```python
from build123d import *

# Parameters (mm, degrees)
F0_R     = 1.9
F0_W     = 19.35
F0_H     = 8
F0_R_2   = 1
F1_DEPTH = 8
F2_R     = 2


with BuildPart() as f1:
    # F0 (on Top) → F1 (new body)
    with BuildSketch(Plane.XY):
        Polygon((50, 22.5), (0, 22.5), (0, 0), (14.45, 0), (33.8, 0), (50, 0), align=None)
        with Locations((7.45, 4.75)):
            Circle(F0_R, mode=Mode.SUBTRACT)
        with Locations((42.5, 17.75)):
            Circle(F0_R, mode=Mode.SUBTRACT)
        with Locations((24.125, -4)):
            Rectangle(F0_W, F0_H)
        with Locations((19.45, -5)):
            Circle(F0_R_2, mode=Mode.SUBTRACT)
        with Locations((28.8, -5)):
            Circle(F0_R_2, mode=Mode.SUBTRACT)
    extrude(amount=F1_DEPTH)

    # F2
    f2_edges = [f1.edges().sort_by_distance(p)[0] for p in [
        (14.45, 0, 4),
        (14.45, -8, 4),
        (33.8, -8, 4),
        (33.8, 0, 4),
        (50, 0, 4),
        (50, 22.5, 4),
        (0, 0, 4),
        (0, 22.5, 4),
    ]]
    fillet(f2_edges, radius=F2_R)


solid = f1.part
```
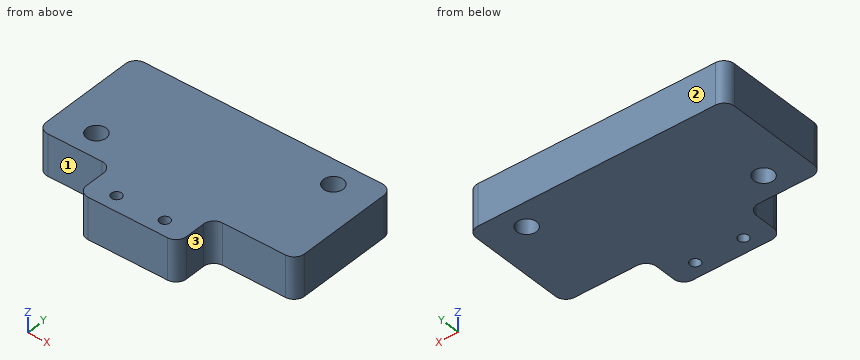
Check sheet for the modelled part. Datum: model origin and axes. Units: mm. Face numbers are marked on the shaded views. A direction names the side the tool comes from. Round coordinates to 2 decimals unless told otherwise and drop trailing zeros. Order: outer loops, then holes, each group sorted by start corner. A loop starts at its lowest first (then second) coordinate and runs counter-clockwise, first axis right, second up.
1) Section check D-D (z = 0.5). Record the boundary of the cut face in (x, y).
2) Section check B-B (x = 19.45). Record the boundary of the cut face in (y, z), and give its area (3 significant figures).
3) Section check A-A (y = -5). Record the boundary of the cut face in (x, z), and give its area (3 significant figures).
4) Section check C-C (y = 4.75). Record the boundary of the cut face in (x, z).
5) Scan lines: line 1 (Y direction, x = 42.5, z = 6.25); line 2 (Y direction, x = 7.5, z = 5); line 3 (Y direction, x = 45, z = 4.5). Record each from-to range of solid material in increasing order.
6) Tool access check on the marked faces 1, 2 and 3. Record the directions out of +Z, -Z, +X, -X, +Y, -Y that give a thin tool (end or side, any length) a straight path to the whole face; none if there is none.
7) Go/stop test with flat-tipped pins: pin 1 Ø3 at (y, z) = (-4.5, 5) entering from -X; pin 2 Ø3.5 at (x, y) = (42.5, 17.75) entering from +Z; pin 3 Ø1.2 at (y, z) = (-3, 6) entering from +X; pin 4 Ø2 at (x, z) = (38, 6) entering from -Y. Record where each tip stops, or that it passes through.
Result:
1. outline: (0, 2) arc R2 ccw to (2, 0) - (12.45, 0) arc R2 cw to (14.45, -2) - (14.45, -6) arc R2 ccw to (16.45, -8) - (31.8, -8) arc R2 ccw to (33.8, -6) - (33.8, -2) arc R2 cw to (35.8, 0) - (48, 0) arc R2 ccw to (50, 2) - (50, 20.5) arc R2 ccw to (48, 22.5) - (2, 22.5) arc R2 ccw to (0, 20.5) - close; hole circle Ø3.8 at (7.45, 4.75); hole circle Ø2 at (19.45, -5); hole circle Ø2 at (28.8, -5); hole circle Ø3.8 at (42.5, 17.75)
2. outline: (-8, 0) - (-6, 0) - (-6, 8) - (-8, 8) - close; (-4, 0) - (22.5, 0) - (22.5, 8) - (-4, 8) - close
2. area: 228 mm2
3. outline: (14.45, 0) - (18.45, 0) - (18.45, 8) - (14.45, 8) - close; (20.45, 0) - (27.8, 0) - (27.8, 8) - (20.45, 8) - close; (29.8, 0) - (33.8, 0) - (33.8, 8) - (29.8, 8) - close
3. area: 123 mm2
4. outline: (0, 0) - (5.55, 0) - (5.55, 8) - (0, 8) - close; (9.35, 0) - (50, 0) - (50, 8) - (9.35, 8) - close
5. line 1: y = 0 to 15.85, 19.65 to 22.5
5. line 2: y = 0 to 2.85, 6.65 to 22.5
5. line 3: y = 0 to 22.5
6. face 1: +Z, -Z, -X, -Y
6. face 2: +Z, -Z, +X, -X, +Y
6. face 3: +Z, -Z, +X, -Y
7. pin 1: stops at x = 14.45
7. pin 2: passes through
7. pin 3: stops at x = 33.8
7. pin 4: stops at y = 0
